from build123d import *

# Parameters (mm, degrees)
SKETCH9_W           = 5.45
SKETCH9_H           = 61.5
BOSS_EXTRUDE3_DEPTH = 8
SKETCH11_W          = 3.5
SKETCH11_H          = 9
CUT_EXTRUDE1_DEPTH  = 63.257148184
SKETCH12_R          = 1.4
BOSS_EXTRUDE4_DEPTH = 5.3
SKETCH13_R          = 1.1
CUT_EXTRUDE2_DEPTH  = 33.212613989
SKETCH14_W          = 4.52927803
SKETCH14_H          = 16
BOSS_EXTRUDE5_DEPTH = 1.5
SKETCH15_W          = 9
SKETCH15_H          = 9
CUT_EXTRUDE3_DEPTH  = 33.237633288


with BuildPart() as part:
    # Sketch9 → Boss-Extrude3 (new, symmetric)
    with BuildSketch(Plane(origin=(0, 0, 0), x_dir=(1, 0, 0), z_dir=(0, 1, 0))):
        with Locations((-2.725, 0)):
            Rectangle(SKETCH9_W, SKETCH9_H)
    extrude(amount=BOSS_EXTRUDE3_DEPTH, both=True)

    # Sketch11 → Cut-Extrude1 (cut, through all)
    with BuildSketch(Plane.XY.offset(30.75)):
        with Locations((-1.75, 0)):
            Rectangle(SKETCH11_W, SKETCH11_H)
    extrude(amount=-CUT_EXTRUDE1_DEPTH, mode=Mode.SUBTRACT)

    # Sketch12 → Boss-Extrude4 (add)
    with BuildSketch(Plane.ZY.offset(5.45)):
        with Locations((-27.45, 2)):
            Circle(SKETCH12_R)
        with Locations((-27.45, -2)):
            Circle(SKETCH12_R)
        with Locations((23.05, 2)):
            Circle(SKETCH12_R)
    extrude(amount=-BOSS_EXTRUDE4_DEPTH)

    # Sketch13 → Cut-Extrude2 (cut, through all)
    with BuildSketch(Plane(origin=(-0.15, 0, 0), x_dir=(0, 0, -1), z_dir=(1, 0, 0))):
        with Locations((-23.05, 2)):
            Circle(SKETCH13_R)
        with Locations((27.45, 2)):
            Circle(SKETCH13_R)
        with Locations((27.45, -2)):
            Circle(SKETCH13_R)
    extrude(amount=-CUT_EXTRUDE2_DEPTH, mode=Mode.SUBTRACT)

    # Sketch14 → Boss-Extrude5 (add)
    with BuildSketch(Plane(origin=(0, 0, -30.75), x_dir=(-1, 0, 0), z_dir=(0, 0, -1))):
        with Locations((2.264639015, 0)):
            Rectangle(SKETCH14_W, SKETCH14_H)
    extrude(amount=-BOSS_EXTRUDE5_DEPTH)

    # Sketch15 → Cut-Extrude3 (cut, through all)
    with BuildSketch(Plane.ZY.offset(5.45)):
        with Locations((3.25, 0)):
            Rectangle(SKETCH15_W, SKETCH15_H)
    extrude(amount=-CUT_EXTRUDE3_DEPTH, mode=Mode.SUBTRACT)


solid = part.part
Model file for the job. Use its own axes, mm. A direction names the side the tool comes from. Give positions to 0.01 mm unless a question says otherwise; leave off trailing zeros. Loops run counter-clockwise (first coordinate to the right, second up) from the corner with the lowest first, then second, coordinate; pieces in that order, holes last. Notation, with made-up numbers: (-26, -38) -> (32, -38) arc R27 ccw to (32, -3) -> close; hole circle Ø4 at (-28, 17.5). An arc over 180 degrees is marked (long way). Use a Markdown table: item, result. Add a question column.
(1) Mould opens along Z. For faces 1 (the cylindrical face through (-2.8, 1.3, 23.9)), 2 (the flat face through (-5.45, 5, 0)), 3 (the flat face through (-4, 0, 30.75)) say: +Z half, -Z half, draft (parallel to the pull), parting line (faces both ways), or undercut.
(2) Slice it at B-B on z = 23.05. List the corners of the cut face in (x, y).
(3) Slice it at D-D on x = -4.75. List the corners of the cut face in (y, z).
(4) Wall check: line 1 along Y through (x, z) = (-1.65, -27.45); line 2 along Y through (x, z) = (-3.1, 23.05); line 3 along Y through (x, z) = (-2.6, 4). Give the ranges that are in metal, low to high.
(5) Tool access for faces 4 (the flat face through (-3, 8, 0)), 5 (the flat face through (-4, 0, -1.25)), 6 (the cylindrical face through (-1.85, 2.06, -28.85)): list every direction of +Z, -Z, +X, -X, +Y, -Y with a clear straight run to the whole face (end or side of a thin tool).
(6) Slice it at A-A on x = -0.8. List the corners of the cut face in (y, z).
(7) Slice it at C-C on y = -2. List the corners of the cut face in (x, z), and give its area (3 significant figures).
(8) Drop flat-ended pins along their axis: pin 1 Ø2 at (y, z) = (1.5, 22.5) entering from +X; pin 2 Ø3 at (x, y) = (-1, 0.5) entering from +Z; pin 3 Ø2.5 at (y, z) = (0, -15) entering from +X; pin 4 Ø2 at (y, z) = (2, -27.45) entering from -X. Give the stop position or say it passes through.
Filled sheet:
| question | item | result |
|---|---|---|
| 1 | face 1 | undercut |
| 1 | face 2 | draft |
| 1 | face 3 | +Z half |
| 2 | outline | (-5.45, -8) -> (0, -8) -> (0, -4.5) -> (-3.5, -4.5) -> (-3.5, 0.6) -> (-0.15, 0.6) -> (-0.15, 0.9) -> (-5.45, 0.9) -> close; (-5.45, 3.1) -> (-0.15, 3.1) -> (-0.15, 3.4) -> (-3.5, 3.4) -> (-3.5, 4.5) -> (0, 4.5) -> (0, 8) -> (-5.45, 8) -> close |
| 3 | outline | (-8, -30.75) -> (8, -30.75) -> (8, 30.75) -> (-8, 30.75) -> close; hole (-4.5, -1.25) -> (4.5, -1.25) -> (4.5, 7.75) -> (-4.5, 7.75) -> close; hole circle Ø2.2 at (-2, -27.45); hole circle Ø2.2 at (2, -27.45); hole circle Ø2.2 at (2, 23.05) |
| 4 | line 1 | -8 to -4.5, -3.4 to -3.1, -0.9 to -0.6, 0.6 to 0.9, 3.1 to 3.4, 4.5 to 8 |
| 4 | line 2 | -8 to -4.5, 0.6 to 0.9, 3.1 to 3.4, 4.5 to 8 |
| 4 | line 3 | -8 to -4.5, 4.5 to 8 |
| 5 | face 4 | +Z, -Z, +X, -X, +Y |
| 5 | face 5 | +X, -X |
| 5 | face 6 | +X |
| 6 | outline | (-8, -30.75) -> (8, -30.75) -> (8, 30.75) -> (4.5, 30.75) -> (4.5, -29.25) -> (-4.5, -29.25) -> (-4.5, 30.75) -> (-8, 30.75) -> close; circle Ø2.8 at (-2, -27.45); circle Ø2.8 at (2, -27.45); circle Ø2.8 at (2, 23.05); hole circle Ø2.2 at (-2, -27.45); hole circle Ø2.2 at (2, -27.45); hole circle Ø2.2 at (2, 23.05) |
| 7 | outline | (-5.45, -30.75) -> (0, -30.75) -> (0, -29.25) -> (-3.5, -29.25) -> (-3.5, -28.85) -> (-0.15, -28.85) -> (-0.15, -28.55) -> (-5.45, -28.55) -> close; (-5.45, -26.35) -> (-0.15, -26.35) -> (-0.15, -26.05) -> (-3.5, -26.05) -> (-3.5, -1.25) -> (-5.45, -1.25) -> close; (-5.45, 7.75) -> (-3.5, 7.75) -> (-3.5, 30.75) -> (-5.45, 30.75) -> close |
| 7 | area | 105 mm2 |
| 8 | pin 1 | x = -0.15 |
| 8 | pin 2 | z = 24.45 |
| 8 | pin 3 | x = -3.5 |
| 8 | pin 4 | through |
